from build123d import *

# Parameters (mm, degrees)
F0_W     = 50.8
F0_H     = 31.75
F1_DEPTH = 25.4
F3_DEPTH = 10.16
F5_DEPTH = 12.7


with BuildPart() as f1:
    # F0 (on Top) → F1 (new body)
    with BuildSketch(Plane.XY):
        with Locations((25.4, 15.875)):
            Rectangle(F0_W, F0_H)
    extrude(amount=F1_DEPTH)

    # F2 (on face) → F3 (join)
    with BuildSketch(Plane.XY.offset(25.4)):
        Polygon((25.4, 31.75), (0, 31.75), (0, 0), (6.35, 0), align=None)
    extrude(amount=F3_DEPTH)

    # F4 (on face) → F5 (join)
    with BuildSketch(Plane.XY.offset(25.4)):
        Polygon((50.8, 15.875), (38.1, 0), (50.8, 0), align=None)
    extrude(amount=F5_DEPTH)


solid = f1.part
The listing builds one solid part. Answer for the finished solid, in the listing's coordinates (mm). A direction names the side the tool comes from. Round coordinates to 2 decimals unless told otherwise and drop trailing zeros. Order: outer loops, then holes, each group sorted by start corner. A loop starts at its lowest first (then second) coordinate and runs counter-clockwise, first axis right, second up. Notation, with made-up numbers: M 43,-34 L 95,-34 A30 cw 95,-3 Z; hole C 89.5,52.5 d8. An arc over 180 degrees is marked long. Answer in a Markdown table with one row per item. Add a question column.
1) Consider line 1 along Z through (x, y) = (37, 7); line 2 along Z through (x, y) = (2, 6.5); line 3 along X through (y, z) = (5, 31). Determine where each line is inside the solid, lowest interval first. Write a range as from..to.
2) Which of the six approach directions +Z, -Z, +X, -X, +Y, -Y give full straight-line access (tool end or side, diameter ignored) to faces 1 (the face through (15.74, 15.65, 30.41)), 2 (the face through (33, 16, 25.4)), 3 (the face through (25, 16, 0)), 4 (the face through (10, 20, 35.56))?
3) The part is cut by section A-A on z = 27.5. Determine the outline of the cut face in (x, y) (3 decimals), plus the area to 3 significant figures.
4) The part is cut by section C-C on x = 8. Determine the outline of the cut face in (y, z), plus the area to 3 significant figures.
5) The part is cut by section B-B on y = 9. Determine the outline of the cut face in (x, z), plus the area to 3 significant figures.
6) Determine the mould class of faces 5 (the face through (0, 16, 18)), 6 (the face through (44.5, 8, 31.7)), 7 (the face through (47, 5, 38.1)) for opening direction X: pulls with the +X half, pulls with the -X half, needs draft (parallel to the pull), parting line crosses it, or undercut.
7) The part is cut by section D-D on y = 27. Determine the outline of the cut face in (x, z).
8) A flat-ended cylindrical pin translates along its axis: pin 1 Ø12 at (x, z) = (17.5, 31.5) entering from -Y. Find the tip coordinate at first contact, or state that the pin passes through.
Findings below:
| question | item | result |
|---|---|---|
| 1 | line 1 | z = 0..25.4 |
| 1 | line 2 | z = 0..35.56 |
| 1 | line 3 | x = 0..9.35, 42.1..50.8 |
| 2 | face 1 | +Z, -Y |
| 2 | face 2 | +Z |
| 2 | face 3 | -Z, +X, -X, +Y, -Y |
| 2 | face 4 | +Z, -X, +Y, -Y |
| 3 | outline | M 0,0 L 6.35,0 L 25.4,31.75 L 0,31.75 Z; M 38.1,0 L 50.8,0 L 50.8,15.875 Z |
| 3 | area | 605 mm² |
| 4 | outline | M 0,0 L 31.75,0 L 31.75,35.56 L 2.75,35.56 L 2.75,25.4 L 0,25.4 Z |
| 4 | area | 1,100 mm² |
| 5 | outline | M 0,0 L 50.8,0 L 50.8,38.1 L 45.3,38.1 L 45.3,25.4 L 11.75,25.4 L 11.75,35.56 L 0,35.56 Z |
| 5 | area | 1,480 mm² |
| 6 | face 5 | pulls with the -X half |
| 6 | face 6 | undercut |
| 6 | face 7 | needs draft |
| 7 | outline | M 0,0 L 50.8,0 L 50.8,25.4 L 22.55,25.4 L 22.55,35.56 L 0,35.56 Z |
| 8 | pin 1 | stops at y = 8.58 |
